The listing builds one solid part. Answer for the finished solid, in the listing's coordinates (mm). Face numbers are marked on the shaded views. A direction names the side the tool comes from. Round coordinates to 2 decimals unless told otherwise and drop trailing zeros. Order: outer loops, then holes, each group sorted by start corner. A loop starts at its lowest first (then second) coordinate and runs counter-clockwise, first axis right, second up. Notation, with made-up numbers: M 74,55.25 L 122,55.25 A9 ccw 122,68.25 Z; hole C -18.75,6 d5. An arc over 180 degrees is marked long. Write item = value, one per line. Start each with the question number.
(1) Which of the six approach directions +Z, -Z, +X, -X, +Y, -Y give full straight-line access (tool end or side, diameter ignored) to the marked faces 1 and 2?
(2) A cutting plane is placed at A-A, the plane x = -4. Determine the outline of the cut face in (y, z).
(3) Each of these flat-tipped pins is pushed along its axis until it touches: pin 1 (1 mm diameter, centred on y = -3, z = 1, fed in from +X); pin 2 (1 mm diameter, centred on x = -11.5, y = 1, fed in from -Z); pin 3 (1.5 mm diameter, centred on x = -17.5, y = 0, fed in from -Z). Where does it stop, or does it pass through?
(4) Straight lines are drawn through the part: probe 1 along Z at (x, y) = (1.5, 2.75); probe 2 along Y at (x, z) = (-4.5, 1.25); probe 3 along Z at (x, y) = (-4.5, 0.5). For each, find the intervals that lie inside material, in ascending order. Write a range as from..to.
(5) For a pull along Z with two mould halves and no side action, classify the marked faces 3, 4 and 5 as released by +Z, released by -Z, zero draft, split by the parting line, or undercut.
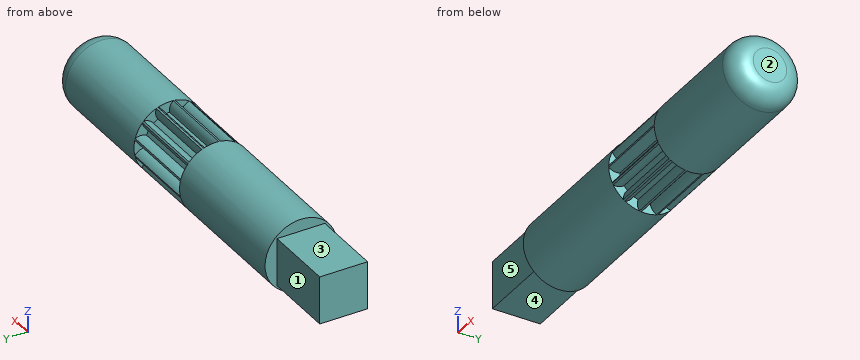
from build123d import *
from build123d.topology import SkipClean

# Parameters (mm, degrees)
BASPROSKE_W         = 8
BASPROSKE_H         = 3.75
TOOTHCUT_DEPTH      = 10.59817691
TEETHCUTS_COUNT     = 13
TEETHCUTS_ANGLE     = 332.307692308
BORSKE_R            = 0.4
BORE_DEPTH          = 50.0000508
SKETCH3_R           = 3.75
BOSS_EXTRUDE3_DEPTH = 15
SKETCH4_W           = 5
SKETCH4_H           = 5
BOSS_EXTRUDE4_DEPTH = 7.5
BOSS_EXTRUDE5_START = 14
SKETCH5_R           = 3.75
BOSS_EXTRUDE5_DEPTH = 14
FILLET1_R           = 2
SKETCH8_R           = 1.303262777
BOSS_EXTRUDE8_DEPTH = 30


with BuildPart() as part:
    # BasProSke → Base-Revolve (revolve)
    with BuildSketch(Plane(origin=(0, 0, 0), x_dir=(1, 0, 0), z_dir=(0, 1, 0)), mode=Mode.PRIVATE) as base_revolve_sk:
        with Locations((4, 1.875)):
            Rectangle(BASPROSKE_W, BASPROSKE_H)
    revolve(base_revolve_sk.sketch.rotate(Axis((-10, 0, 0), (1, 0, 0)), 180), axis=Axis((-10, 0, 0), (1, 0, 0)))

    # TooCutSke → ToothCut (cut, through all)
    with BuildSketch(Plane(origin=(0, 0, 0), x_dir=(0, 0, -1), z_dir=(1, 0, 0))):
        with BuildLine():
            ThreePointArc((0.275247387, 2.609523879), (0, 2.624), (-0.275247387, 2.609523879))
            ThreePointArc((-0.275247387, 2.609523879), (-0.421084752, 3.214694797), (-0.831556081, 3.682683756))
            ThreePointArc((-0.831556081, 3.682683756), (0, 3.7754), (0.831556081, 3.682683756))
            ThreePointArc((0.831556081, 3.682683756), (0.421084752, 3.214694797), (0.275247387, 2.609523879))
        make_face()
    toothcut = extrude(amount=TOOTHCUT_DEPTH, mode=Mode.SUBTRACT)

    # TeethCuts: ToothCut ×13 about axis
    teethcuts_axis = Axis((-10, 0, 0), (1, 0, 0))
    for i in range(1, TEETHCUTS_COUNT):
        add(toothcut.rotate(teethcuts_axis, i * TEETHCUTS_ANGLE / (TEETHCUTS_COUNT - 1)), mode=Mode.SUBTRACT)

    # BorSke → Bore (cut, symmetric)
    with BuildSketch(Plane(origin=(0, 0, 0), x_dir=(0, 0, -1), z_dir=(1, 0, 0))):
        with Locations(Location((0, 0, 0), (0, 0, 180))):
            Circle(BORSKE_R)
    extrude(amount=BORE_DEPTH, both=True, mode=Mode.SUBTRACT)

    # Sketch3 → Boss-Extrude3 (add)
    with SkipClean():  # the faces are left unmerged after this step: merging them gives an invalid solid
        with BuildSketch(Plane.ZY):
            Circle(SKETCH3_R)
        extrude(amount=BOSS_EXTRUDE3_DEPTH)

    # Sketch4 → Boss-Extrude4 (add)
    with SkipClean():  # the faces are left unmerged after this step: merging them gives an invalid solid
        with BuildSketch(Plane.ZY.offset(15)):
            Rectangle(SKETCH4_W, SKETCH4_H)
        extrude(amount=BOSS_EXTRUDE4_DEPTH)

    # Sketch5 → Boss-Extrude5 (add)
    with BuildSketch(Plane(origin=(8, 0, 0), x_dir=(0, 0, -1), z_dir=(1, 0, 0)).offset(BOSS_EXTRUDE5_START)):
        with Locations(Location((0, 0, 0), (0, 0, 180))):
            Circle(SKETCH5_R)
    extrude(amount=-BOSS_EXTRUDE5_DEPTH)

    # Fillet1
    fillet1_edges = [part.edges().sort_by_distance(p)[0] for p in [
        (22, 0, -3.75),
    ]]
    fillet(fillet1_edges, radius=FILLET1_R)

    # Sketch8 → Boss-Extrude8 (add)
    with BuildSketch(Plane(origin=(22, 0, 0), x_dir=(0, 0, -1), z_dir=(1, 0, 0))):
        Circle(SKETCH8_R)
    extrude(amount=-BOSS_EXTRUDE8_DEPTH)


solid = part.part
Reported:
q1.face_1 = +Z, -Z, -X, +Y
q1.face_2 = +Z, -Z, +X, +Y, -Y
q2.outline = C 0,0 d7.5
q3.pin_1 = 21.78
q3.pin_2 = -3.72
q3.pin_3 = -2.5
q4.probe_1 = -2.55..-2.03, -1.09..-0.28, 0.28..1.09, 2.03..2.55
q4.probe_2 = -3.54..3.54
q4.probe_3 = -3.72..3.72
q5.face_3 = released by +Z
q5.face_4 = released by -Z
q5.face_5 = zero draft
